Model file for the job. Use its own axes, mm. Face numbers are marked on the shaded views. A direction names the side the tool comes from. Coordinates: 2 decimals unless noted, no trailing zeros. Order: outer loops, then holes, each group sorted by start corner. A loop starts at its lowest first (then second) coordinate and runs counter-clockwise, first axis right, second up. Notation, with made-up numbers: M 8,28 L 57,28 A27 ccw 57,53 Z; hole C -35,87 d3. An arc over 180 degrees is marked long. Return JSON: item names as keys, results as strings.
Autodesk Inventor part; units mm, degrees
ref_plane "YZ Plane" through (0, 0, 0) normal (1, 0, 0) x (0, 1, 0)
ref_plane "XZ Plane" through (0, 0, 0) normal (0, 1, 0) x (-1, 0, 0)
ref_plane "XY Plane" through (0, 0, 0) normal (0, 0, 1) x (1, 0, 0)
sketch "Sketch1" plane through (0, 0, 0) normal (0, 0, 1) x (1, 0, 0)
  circle A0 centre (-16, 0) radius 1
  circle A1 centre (-13, 0) radius 1
  circle A2 centre (0, 0) radius 1.5
  arc A3 (-19.2347, 2.9908) -> (-19.2347, -2.9908) centre (-19, 0) ccw
  arc A4 (-0.7018, -4.4449) -> (-0.7018, 4.4449) centre (0, 0) ccw
  line L0 (0, -4.5) -> (-19.2347, -2.9908)
  line L1 (0, 4.5) -> (-19.2347, 2.9908)
  dimension "d1" = 2
  dimension "d2" = 2
  dimension "d3" = 3
  dimension "d6" = 3
  dimension "d8" = 6
  dimension "d9" = 9
  dimension "d10" = 3
extrude "Extrusion1" add sketch "Sketch1" along normal blind 2 contours L1 A4 L0 A3
sketch "Sketch2" plane through (0, 0, 2) normal (0, 0, 1) x (1, 0, 0)
  circle A0 centre (0, 0) radius 1.5
  arc A1 (0, -4.5) -> (0, 4.5) centre (0, 0) ccw
  circle A2 centre (0, 0) radius 4.5
  dimension "d13" = 9
extrude "Extrusion2" add sketch "Sketch2" along normal blind 2
sketch "Sketch3" plane through (0, 0, 4) normal (0, 0, 1) x (1, 0, 0)
  circle A0 centre (0, 0) radius 1.5
  circle A1 centre (0, 0) radius 4.5
  circle A2 centre (0, 0) radius 2.5
  dimension "d16" = 5
hole "Hole1" at (0, 0, 4) direction (0, 0, -1) diameter 5 depth 2
sketch "Sketch4" plane through (0, 0, 2) normal (0, 0, 1) x (1, 0, 0)
  arc A0 (-19.2347, 2.9908) -> (-19.2347, -2.9908) centre (-19, 0) ccw
  circle A1 centre (-16, 0) radius 1
  circle A2 centre (-13, 0) radius 1
  circle A3 centre (-19, 0) radius 1
  circle A4 centre (-10, 0) radius 1
  dimension "d24" = 2
  dimension "d25" = 2
  dimension "d26" = 3
  dimension "d27" = 3
hole "Hole2" at (-19, 0, 2) at (-10, 0, 2) direction (0, 0, -1) diameter 2 end through all
properties part number "horn aluminium"
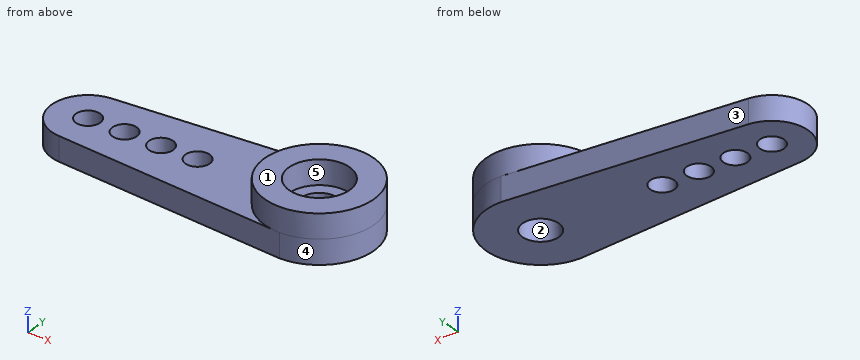
Item 1: 3-axis set-ups, long thin cutter, end or side, ignore diameter. For the marked faces 4 and 5: which of +Z, -Z, +X, -X, +Y, -Y reach the whole face in a straight line?
Check result:
{"face 4": "+Z, -Z, +X", "face 5": "+Z"}
Item 2: Saw through at B-B (y = -0.75). Count the separate pieces of the cut face and the enclosed holes in it, and give its area (3 significant figures).
Check result:
{"separate pieces": "6", "enclosed holes": "0", "area": "45.1 mm2"}
Item 3: Saw through at A-A (x = -19). Write the cut outline in (y, z), and give its area (3 significant figures).
Check result:
{"outline": "M -3.01,0 L -1,0 L -1,2 L -3.01,2 Z; M 1,0 L 3.01,0 L 3.01,2 L 1,2 Z", "area": "8.04 mm2"}
Item 4: Drop flat-ended pins along their axis: pin 1 Ø4 at (x, y) = (-17.5, 3) entering from -Z; pin 2 Ø5 at (x, y) = (-19, 1) entering from +Z; pin 3 Ø1.6 at (x, y) = (-16, 0) entering from +Z; pin 4 Ø1 at (x, z) = (-4.5, 0.5) entering from -Y. Give the stop position or say it passes through.
Check result:
{"pin 1": "stops at z = 0", "pin 2": "stops at z = 2", "pin 3": "passes through", "pin 4": "stops at y = -4.19"}
Item 5: Pull direction X, two halves, no side cores. Call the marked faces 1, 2 and 3: +X half, -X half, draft (parallel to the pull), parting line (faces both ways), or undercut.
Check result:
{"face 1": "draft", "face 2": "undercut", "face 3": "-X half"}
Item 6: Wall check: line 1 (Y direction, x = -10, z = 0.85); line 2 (Z direction, x = -7, y = -1); line 3 (X direction, y = -1.5, z = 3.6). Give the ranges that are in metal, low to high.
Check result:
{"line 1": "y = -3.72 to -1, 1 to 3.72", "line 2": "z = 0 to 2", "line 3": "x = -4.24 to -2, 2 to 4.24"}
Item 7: Saw through at C-C (z = 0.9). Write the cut outline in (x, y).
Check result:
{"outline": "M -19.23,-2.99 L 0,-4.5 A4.5 ccw 0,4.5 L -19.23,2.99 A3 ccw Z; hole C -19,0 d2; hole C -16,0 d2; hole C -13,0 d2; hole C -10,0 d2; hole C 0,0 d3"}
